The listing builds one solid part. Answer for the finished solid, in the listing's coordinates (mm). Face numbers are marked on the shaded views. A direction names the side the tool comes from. Coordinates: 2 decimals unless noted, no trailing zeros. Order: outer loops, then holes, each group sorted by start corner. A loop starts at its lowest first (then second) coordinate and runs counter-clockwise, first axis right, second up. Notation, with made-up numbers: (-24, 7) - (-18, 7) arc R21 ccw to (-18, 35) - close; hole circle Ø5 at (69.25, 88.5). An arc over 180 degrees is marked (long way). One line per item, written item: value. Start each with the question number.
```python
from build123d import *

# Parameters (mm, degrees)
SKETCH1_W            = 24
SKETCH1_H            = 12
EXTRUDE1_DEPTH       = 21.5
SKETCH2_W            = 3.43
SKETCH2_H            = 12
EXTRUDE2_DEPTH       = 4.318
FILLET1_R            = 2
FILLET2_R            = 2
SKETCH3_R            = 1.016
CUT_EXTRUDE1_DEPTH   = 4.318
FILLET1_OF_MIRROR1_R = 2
FILLET2_OF_MIRROR1_R = 2
SKETCH4_R            = 6.02
EXTRUDE3_DEPTH       = 4.725


with BuildPart() as part:
    # Sketch1 → Extrude1 (new body)
    with BuildSketch(Plane.XY):
        with Locations((-12, 6)):
            Rectangle(SKETCH1_W, SKETCH1_H)
    extrude(amount=EXTRUDE1_DEPTH)

    # Sketch2 → Extrude2 (add)
    with BuildSketch(Plane.ZY.offset(24)):
        with Locations((18.715, 6)):
            Rectangle(SKETCH2_W, SKETCH2_H)
    extrude2 = extrude(amount=EXTRUDE2_DEPTH)

    # Fillet1
    fillet1_edges = [part.edges().sort_by_distance(p)[0] for p in [
        (-28.318, 12, 18.715),
    ]]
    fillet(fillet1_edges, radius=FILLET1_R)

    # Fillet2
    fillet2_edges = [part.edges().sort_by_distance(p)[0] for p in [
        (-28.318, 0, 18.715),
    ]]
    fillet(fillet2_edges, radius=FILLET2_R)

    # Sketch3 → Cut-Extrude1 (cut)
    with BuildSketch(Plane.XY.offset(20.43)):
        with Locations((-25.778, 2.53620247)):
            Circle(SKETCH3_R)
        with Locations((-25.778, 9.46)):
            Circle(SKETCH3_R)
    cut_extrude1 = extrude(amount=-CUT_EXTRUDE1_DEPTH, mode=Mode.SUBTRACT)

    # Mirror1: Extrude2, Cut-Extrude1 across plane
    add(extrude2.mirror(Plane.ZY.offset(12)))
    add(cut_extrude1.mirror(Plane.ZY.offset(12)), mode=Mode.SUBTRACT)

    # Fillet1 of Mirror1
    fillet1_of_mirror1_edges = [part.edges().sort_by_distance(p)[0] for p in [
        (4.318, 12, 18.715),
    ]]
    fillet(fillet1_of_mirror1_edges, radius=FILLET1_OF_MIRROR1_R)

    # Fillet2 of Mirror1
    fillet2_of_mirror1_edges = [part.edges().sort_by_distance(p)[0] for p in [
        (4.318, 0, 18.715),
    ]]
    fillet(fillet2_of_mirror1_edges, radius=FILLET2_OF_MIRROR1_R)

    # Sketch4 → Extrude3 (add)
    with BuildSketch(Plane.XY.offset(21.5)):
        with Locations(Location((-17.98, 5.987133141, 0), (0, 0, 180))):
            Circle(SKETCH4_R)
    extrude(amount=EXTRUDE3_DEPTH)


solid = part.part
```
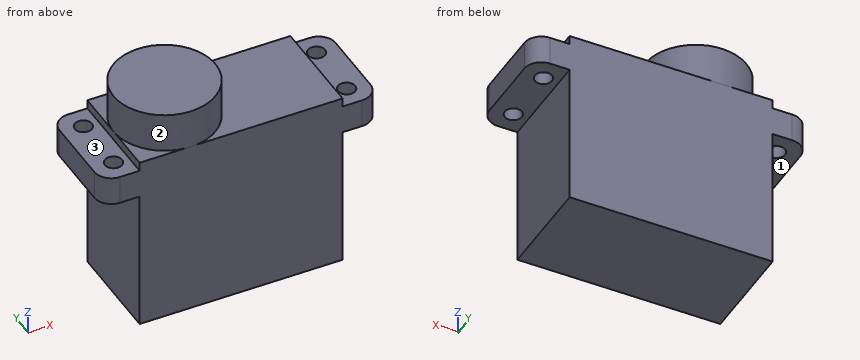
(1) The part is cut by section C-C on y = 7. Determine the outline of the cut face in (x, z) (3 decimals), plus the area to 3 significant figures.
(2) The part is cut by section D-D on z = 14.25. Determine the outline of the cut face in (x, y), plus the area to 3 significant figures.
(3) The part is cut by section A-A on y = 9.46. Determine the outline of the cut face in (x, z) (3 decimals), plus the area to 3 significant figures.
(4) Consider probe 1 along X at (y, z) = (10.25, 18); probe 2 along Y at (x, z) = (-15.5, 6.75); probe 3 along X at (y, z) = (6.5, 9.5). Determine where each line is inside the solid, lowest interval first.
(5) For the marked faces 1, 2 and 3, determine the directions among +Z, -Z, +X, -X, +Y, -Y from which every point of the face is accessible in a straight line to the end or side of a thin tool.
(6) The part is cut by section B-B on x = -8. Determine the outline of the cut face in (y, z), plus the area to 3 significant figures.
(7) Flat-ended cylindrical pins translate along their axes: pin 1 Ø12 at (x, z) = (-7.5, 7) entering from +Y; pin 2 Ø1.3 at (x, y) = (-26, 8.5) entering from -Z; pin 3 Ø4.5 at (x, y) = (2.5, 4) entering from +Z. Find the tip coordinate at first contact, or state that the pin passes through.
Completed:
1. outline: (-28.318, 17) - (-24, 17) - (-24, 0) - (0, 0) - (0, 17) - (4.318, 17) - (4.318, 20.43) - (0, 20.43) - (0, 21.5) - (-12.046, 21.5) - (-12.046, 26.225) - (-23.914, 26.225) - (-23.914, 21.5) - (-24, 21.5) - (-24, 20.43) - (-28.318, 20.43) - close
1. area: 602 mm2
2. outline: (-24, 0) - (0, 0) - (0, 12) - (-24, 12) - close
2. area: 288 mm2
3. outline: (-28.318, 17) - (-26.794, 17) - (-26.794, 20.43) - (-28.318, 20.43) - close; (-24.762, 17) - (-24, 17) - (-24, 0) - (0, 0) - (0, 17) - (0.762, 17) - (0.762, 20.43) - (0, 20.43) - (0, 21.5) - (-13.063, 21.5) - (-13.063, 26.225) - (-22.897, 26.225) - (-22.897, 21.5) - (-24, 21.5) - (-24, 20.43) - (-24.762, 20.43) - close; (2.794, 17) - (4.318, 17) - (4.318, 20.43) - (2.794, 20.43) - close
3. area: 578 mm2
4. probe 1: x = -28.3 to -26.42, -25.14 to 1.14, 2.42 to 4.3
4. probe 2: y = 0 to 12
4. probe 3: x = -24 to 0
5. face 1: -Z, -X, +Y, -Y
5. face 2: +Z
5. face 3: +Z, -X, +Y, -Y
6. outline: (0, 0) - (12, 0) - (12, 21.5) - (0, 21.5) - close
6. area: 258 mm2
7. pin 1: stops at y = 12
7. pin 2: stops at z = 17
7. pin 3: stops at z = 20.43
